from build123d import *

# Parameters (mm, degrees)
BOSS_EXTRUDE1_DEPTH = 4
SKETCH4_W           = 21.88
SKETCH4_H           = 53
SKETCH4_R           = 5
CUT_EXTRUDE1_DEPTH  = 4


with BuildPart() as part:
    # Layer1 → Boss-Extrude1 (new body)
    with BuildSketch(Plane(origin=(0, 0, 0), x_dir=(1, 0, 0), z_dir=(0, 1, 0))):
        with BuildLine():
            Line((27, 42), (11.25, 42))
            Line((11.25, 42), (11.25, 24))
            Line((11.25, 24), (-11.25, 24))
            Line((-11.25, 24), (-11.25, 42))
            Line((-11.25, 42), (-27, 42))
            ThreePointArc((-27, 42), (-37.606601718, 37.606601718), (-42, 27))
            Line((-42, 27), (-42, 21.5))
            Line((-42, 21.5), (-42, -21.5))
            Line((-42, -21.5), (-42, -27))
            ThreePointArc((-42, -27), (-37.606601718, -37.606601718), (-27, -42))
            Line((-27, -42), (-11.25, -42))
            Line((-11.25, -42), (-11.25, -24))
            Line((-11.25, -24), (11.25, -24))
            Line((11.25, -24), (11.25, -42))
            Line((11.25, -42), (27, -42))
            ThreePointArc((27, -42), (37.606601718, -37.606601718), (42, -27))
            Line((42, -27), (42, 27))
            ThreePointArc((42, 27), (37.606601718, 37.606601718), (27, 42))
        make_face()
    extrude(amount=BOSS_EXTRUDE1_DEPTH)

    # Sketch4 → Cut-Extrude1 (cut)
    with BuildSketch(Plane(origin=(0, 4, 0), x_dir=(1, 0, 0), z_dir=(0, 1, 0))):
        with Locations((31.06, 0)):
            Rectangle(SKETCH4_W, SKETCH4_H)
        with Locations((32, 32)):
            Circle(SKETCH4_R)
        with Locations((-32, 32)):
            Circle(SKETCH4_R)
        with Locations((-32, -32)):
            Circle(SKETCH4_R)
        with Locations((32, -32)):
            Circle(SKETCH4_R)
    extrude(amount=-CUT_EXTRUDE1_DEPTH, mode=Mode.SUBTRACT)


solid = part.part
Geometry: final body of the model. Coordinates: model frame, mm. A direction names the side the tool comes from. Give positions to 0.01 mm unless a question says otherwise; leave off trailing zeros. Order: outer loops, then holes, each group sorted by start corner. A loop starts at its lowest first (then second) coordinate and runs counter-clockwise, first axis right, second up. Notation, with made-up numbers: (21, 70) -> (65, 70) arc R7 cw to (65, 75) -> close; hole circle Ø1 at (84.5, -32.5). An arc over 180 degrees is marked (long way). Write each question's results on one line, items separated by ' | '.
1) First-contact query: pin 1 Ø2 at (y, z) = (2.5, 35) entering from -X; pin 2 Ø2 at (y, z) = (1.5, -33.5) entering from +X; pin 3 Ø1.2 at (y, z) = (2.5, 1) entering from +X. Flat tips, straight axial feed; report the tip coordinate or a pass-through.
Geometry says:
pin 1: stops at x = -40.27 | pin 2: stops at x = 40.96 | pin 3: stops at x = 20.12
2) Cut plane A-A (x = 36). Output: boundary loops of the cut face in (y, z), and give its area (3 significant figures).
Geometry says:
outline: (0, -39) -> (4, -39) -> (4, -35) -> (0, -35) -> close; (0, -29) -> (4, -29) -> (4, -26.5) -> (0, -26.5) -> close; (0, 26.5) -> (4, 26.5) -> (4, 29) -> (0, 29) -> close; (0, 35) -> (4, 35) -> (4, 39) -> (0, 39) -> close | area: 52.0 mm²
3) Line query: line 1 along X through (y, z) = (2.4, -32); line 2 along X through (y, z) = (0.7, 36); line 3 along Z through (x, y) = (20.5, 2.35). Output: solid intervals per line, ascending.
Geometry says:
line 1: x = -41.14 to -37, -27 to -11.25, 11.25 to 27, 37 to 41.14 | line 2: x = -39 to -35, -29 to -11.25, 11.25 to 29, 35 to 39 | line 3: z = -42 to -26.5, 26.5 to 42
4) Cut plane B-B (y = 1.35). Output: boundary loops of the cut face in (x, z).
Geometry says:
outline: (-42, -27) arc R15 ccw to (-27, -42) -> (-11.25, -42) -> (-11.25, -24) -> (11.25, -24) -> (11.25, -42) -> (27, -42) arc R15 ccw to (42, -27) -> (42, -26.5) -> (20.12, -26.5) -> (20.12, 26.5) -> (42, 26.5) -> (42, 27) arc R15 ccw to (27, 42) -> (11.25, 42) -> (11.25, 24) -> (-11.25, 24) -> (-11.25, 42) -> (-27, 42) arc R15 ccw to (-42, 27) -> close; hole circle Ø10 at (-32, -32); hole circle Ø10 at (-32, 32); hole circle Ø10 at (32, -32); hole circle Ø10 at (32, 32)
5) Cut plane D-D (x = -32). Output: boundary loops of the cut face in (y, z).
Geometry says:
outline: (0, -41.14) -> (4, -41.14) -> (4, -37) -> (0, -37) -> close; (0, -27) -> (4, -27) -> (4, 27) -> (0, 27) -> close; (0, 37) -> (4, 37) -> (4, 41.14) -> (0, 41.14) -> close
6) Draft query along Z for faces 1 (the face through (-37.72, 1.97, 37.49)), 2 (the face through (37.72, 1.97, -37.49)), 3 (the face through (27, 2, -32)), 4 (the face through (27, 2, 32)). Return one class per face: released by +Z, released by -Z, zero draft, split by the parting line, or undercut.
Geometry says:
face 1: released by +Z | face 2: released by -Z | face 3: undercut | face 4: undercut
7) Set-up query: faces 5 (the face through (31, 2, -26.5)), 6 (the face through (-37.49, 1.97, -37.72)), 7 (the face through (-11.25, 2, -33)), 8 (the face through (11.25, 2, 33)). Return all of +Z, -Z, +X, -X, +Y, -Y with unobstructed straight access to the full face (end or side cutting, diameter ignored); none if empty.
Geometry says:
face 5: +X, +Y, -Y | face 6: -Z, -X, +Y, -Y | face 7: -Z, +Y, -Y | face 8: +Z, +Y, -Y
8) Cut plane C-C (z = 30). Output: boundary loops of the cut face in (x, y), and give its area (3 significant figures).
Geometry says:
outline: (-41.7, 0) -> (-36.58, 0) -> (-36.58, 4) -> (-41.7, 4) -> close; (-27.42, 0) -> (-11.25, 0) -> (-11.25, 4) -> (-27.42, 4) -> close; (11.25, 0) -> (27.42, 0) -> (27.42, 4) -> (11.25, 4) -> close; (36.58, 0) -> (41.7, 0) -> (41.7, 4) -> (36.58, 4) -> close | area: 170 mm²
